from build123d import *

# Parameters (mm, degrees)
F0_R     = 4.75
F0_R_2   = 2.25
F1_DEPTH = 3
F2_DEPTH = 2
F3_SIZE  = 0.5


with BuildPart() as f1:
    # F0 (on Top) → F1 (new body)
    with BuildSketch(Plane.XY):
        Circle(F0_R)
        Circle(F0_R_2, mode=Mode.SUBTRACT)
    extrude(amount=F1_DEPTH)

    # F0 (on Top) → F2 (join)
    with BuildSketch(Plane.XY):
        Circle(F0_R)
        Circle(F0_R_2, mode=Mode.SUBTRACT)
        Circle(F0_R_2)
    extrude(amount=-F2_DEPTH)

    # F3
    f3_edges = [f1.edges().sort_by_distance(p)[0] for p in [
        (-4.75, 0, 3),
        (-4.75, 0, -2),
    ]]
    chamfer(f3_edges, length=F3_SIZE)


solid = f1.part
CAD build for the part. Positions are in the model's coordinates, mm. A direction names the side the tool comes from. Round coordinates to 2 decimals unless told otherwise and drop trailing zeros. Order: outer loops, then holes, each group sorted by start corner. A loop starts at its lowest first (then second) coordinate and runs counter-clockwise, first axis right, second up. Notation, with made-up numbers: (0.25, -32.75) - (23.25, -32.75) arc R29 ccw to (23.25, -12.75) - close; hole circle Ø10 at (42.25, 29.25). An arc over 180 degrees is marked (long way). Return JSON: item names as keys, results as strings.
(1) Wall check: probe 1 along Y at (x, z) = (0, 0.8); probe 2 along X at (y, z) = (-2, 0.5); probe 3 along Z at (x, y) = (-0.5, -1.5). Give the ranges that are in metal, low to high. Write a range as from..to.
Answer key:
{"probe 1": "y = -4.75..-2.25, 2.25..4.75", "probe 2": "x = -4.31..-1.03, 1.03..4.31", "probe 3": "z = -2..0"}
(2) Pin check, flat tips, straight feed: pin 1 Ø1.3 at (x, y) = (0, -1) entering from +Z; pin 2 Ø1.5 at (y, z) = (-1, -1) entering from +X; pin 3 Ø3 at (x, z) = (-2, 0) entering from -Y. Stop position of each tip, or through.
Answer key:
{"pin 1": "stops at z = 0", "pin 2": "stops at x = 4.74", "pin 3": "stops at y = -4.72"}
(3) Cut at A-A (y = 0). Give the cut face in (x, z).
Answer key:
{"outline": "(-4.75, -1.5) - (-4.25, -2) - (4.25, -2) - (4.75, -1.5) - (4.75, 2.5) - (4.25, 3) - (2.25, 3) - (2.25, 0) - (-2.25, 0) - (-2.25, 3) - (-4.25, 3) - (-4.75, 2.5) - close"}
(4) Tool access for faces 4 (the face through (-0.29, 2.23, 1.48)), 5 (the face through (0, 0, -2)): list every direction of +Z, -Z, +X, -X, +Y, -Y with a clear straight run to the whole face (end or side of a thin tool).
Answer key:
{"face 4": "+Z", "face 5": "-Z, +X, -X, +Y, -Y"}
(5) Pull direction X, two halves, no side cores. Call faces 1 (the face through (0, 0, 0)), 2 (the face through (2, -2, 3)), 3 (the face through (2.192, -4.214, 0.528)): +X half, -X half, draft (parallel to the pull), parting line (faces both ways), or undercut.
Answer key:
{"face 1": "undercut", "face 2": "draft", "face 3": "parting line"}
(6) Cut at C-C (z = 2.2). Give the cut face in (x, y).
Answer key:
{"outline": "circle Ø9.5 at (0, 0); hole circle Ø4.5 at (0, 0)"}
(7) Cut at D-D (z = -0.85). Give the cut face in (x, y), then the cut area to 3 significant figures.
Answer key:
{"outline": "circle Ø9.5 at (0, 0)", "area": "70.9 mm^2"}
